The figure shows three views and two pictorial views of one solid part (mm, origin at its lowest corner). Answer the questions. A direction names the side the tool comes from. Coordinates: 2 decimals unless noted, no trailing zeros. Loops run counter-clockwise (first coordinate to the right, second up) from the corner with the lowest first, then second, coordinate; pieces in that order, holes last. Notation, with made-up numbers: (-28.5, 47.5) -> (-21.5, 47.5) arc R10 ccw to (-21.5, 57.5) -> close; hole circle Ø4 at (5, -7.5). An arc over 180 degrees is marked (long way). Answer as a JSON object with one key per item and string values. Group by question number.
1) Flat-ended cylindrical pins translate along their axes: P1, Ø5, axis at x = 10, z = 21.5, coming from the -Y side; P2, Ø5.5, axis at y = 6, z = 11.5, coming from the +X side. Find the tip coordinate at first contact, or state that the pin passes through.
2) Section B-B, the plane y = 8 is taken. Give the vertices of the cut face in (x, z), plus the area to 3 significant figures.
3) Consider probe 1 along Y at (x, z) = (15.5, 26.25); probe 2 along X at (y, z) = (9, 7.5); probe 3 along X at (y, z) = (19.75, 2.5). Determine where each line is inside the solid, lowest interval first. Write a range as [from, to].
4) Section A-A, the plane z = 22.5 is taken. Give the vertices of the cut face in (x, y).
5) Section C-C, the plane x = 16.75 is taken. Give the vertices of the cut face in (y, z).
6) Which of the six approach directions +Z, -Z, +X, -X, +Y, -Y give full straight-line access (tool end or side, diameter ignored) to the marked faces 1 and 2?
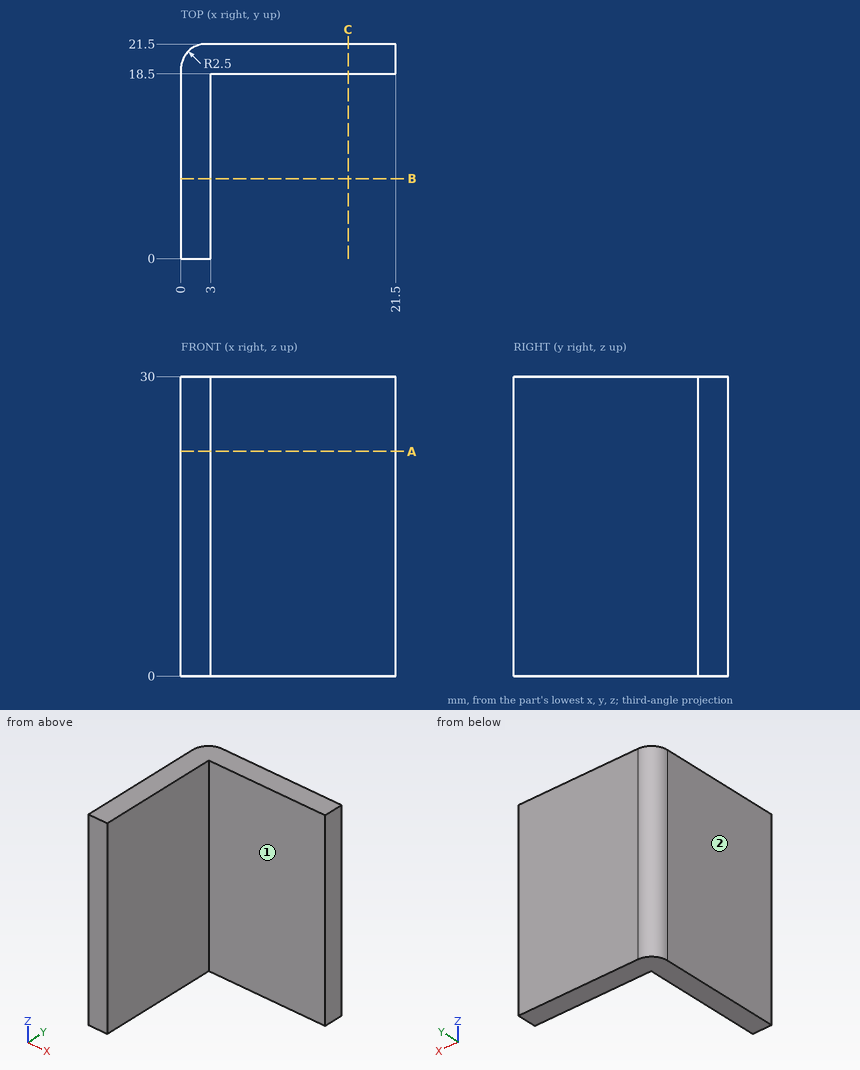
Determined:
{
 "1": {"P1": "y = 18.5", "P2": "x = 3"},
 "2": {"outline": "(0, 0) -> (3, 0) -> (3, 30) -> (0, 30) -> close", "area": "90.0 mm²"},
 "3": {"probe 1": "[18.5, 21.5]", "probe 2": "[0, 3]", "probe 3": "[0.12, 21.5]"},
 "4": {"outline": "(0, 0) -> (3, 0) -> (3, 18.5) -> (21.5, 18.5) -> (21.5, 21.5) -> (2.5, 21.5) arc R2.5 ccw to (0, 19) -> close"},
 "5": {"outline": "(18.5, 0) -> (21.5, 0) -> (21.5, 30) -> (18.5, 30) -> close"},
 "6": {"face 1": "+Z, -Z, +X, -Y", "face 2": "+Z, -Z, -X, +Y, -Y"}
}
